Source: CAD feature listing. Evaluate the final solid. Frame: model axes, mm. A direction names the side the tool comes from. Give positions to 0.01 mm unless a question says otherwise; leave off trailing zeros. Write each loop counter-clockwise with the first axis right and the second up, starting at its lowest first coordinate (ties: lowest second). Pieces come first, ordered by that corner, then holes. Notation, with made-up numbers: (-34.75, 9.5) - (-25.75, 9.5) arc R14 cw to (-25.75, 30.5) - close; hole circle Ø5 at (53, 68). An arc over 180 degrees is marked (long way). One line per question, with ' | ' between items. Start each with the question number.
(1) Section D-D, the plane z = -3.6. Return loops of the section in (x, y) (1 decimal).
(2) Pin query (flat end, axial travel): pin 1 (1.4 mm diameter, centred on x = 6.73, y = -165.72, fed in from -Z); pin 2 (2 mm diameter, centred on y = -165.5, z = -1.5, fed in from +X); pin 3 (3 mm diameter, centred on y = -164, z = 0.5, fed in from -X). Return the tip coordinate at first contact, or that it passes through.
(3) Access query for faces 1 (the cylindrical face through (3.69, -162.93, -2)), 2 (the flat face through (7, -167, 1.588)). Directions: +Z, -Z, +X, -X, +Y, -Y. A direction counts if a zero-diameter tool reaches every point of the face in a straight line with its end or side. Return the directions, or none.
(4) Section A-A, the plane y = -166. Return loops of the section in (x, z).
(5) Section C-C, the plane x = 9.25. Return loops of the section in (y, z).
(6) Ray query, line 1 (Z direction, x = 11.25, y = -166.5); line 2 (Y direction, x = 7.5, z = -0.7); line 3 (Y direction, x = 7.5, z = 1.05). Return the intervals inside material, ascending. Write a range as [from, to].
(7) Section B-B, the plane y = -167.5. Return loops of the section in (x, z).
```python
from build123d import *

# Parameters (mm, degrees)
SKETCH1_R                    = 4.1275
BOSS_EXTRUDE2_DEPTH          = 4.064
SKETCH2_R                    = 4.8895
BOSS_EXTRUDE3_DEPTH          = 1.5875
F_56_0_0465_DIAMETER_HOLE1_D = 1.1811


with BuildPart() as part:
    # Sketch1 → Boss-Extrude2 (new body)
    with BuildSketch(Plane.XY):
        with Locations((6.731, -165.7192297)):
            Circle(SKETCH1_R)
    extrude(amount=-BOSS_EXTRUDE2_DEPTH)

    # Sketch2 → Boss-Extrude3 (add)
    with BuildSketch(Plane.XY):
        with Locations((6.731, -165.7192297)):
            Circle(SKETCH2_R)
    extrude(amount=BOSS_EXTRUDE3_DEPTH)

    # #56 (0.0465) Diameter Hole1 (through all)
    with Locations(Plane(origin=(0, 0, -4.064), x_dir=(-1, 0, 0), z_dir=(0, 0, -1))):
        with Locations((-6.731, -165.7192297)):
            Hole(F_56_0_0465_DIAMETER_HOLE1_D / 2)


solid = part.part
```
Check sheet entries:
1) outline: circle Ø8.3 at (6.7, -165.7); hole circle Ø1.2 at (6.7, -165.7)
2) pin 1: z = -4.06 | pin 2: x = 10.86 | pin 3: x = 1.85
3) face 1: -Z | face 2: +Z, +X, -X, +Y, -Y
4) outline: (1.85, 0) - (2.61, 0) - (2.61, -4.06) - (6.21, -4.06) - (6.21, 1.59) - (1.85, 1.59) - close; (7.25, -4.06) - (10.85, -4.06) - (10.85, 0) - (11.61, 0) - (11.61, 1.59) - (7.25, 1.59) - close
5) outline: (-169.91, 0) - (-168.99, 0) - (-168.99, -4.06) - (-162.45, -4.06) - (-162.45, 0) - (-161.53, 0) - (-161.53, 1.59) - (-169.91, 1.59) - close
6) line 1: [0, 1.59] | line 2: [-169.77, -161.66] | line 3: [-170.55, -160.89]
7) outline: (2.18, 0) - (3.01, 0) - (3.01, -4.06) - (10.45, -4.06) - (10.45, 0) - (11.28, 0) - (11.28, 1.59) - (2.18, 1.59) - close
